```python
from build123d import *

# Parameters (mm, degrees)
SKETCH2_R           = 3.142219065
SKETCH2_W           = 25.3952265
SKETCH2_H           = 12.629529533
SKETCH2_R_2         = 3.175
SKETCH2_R_3         = 8.75000028
BOSS_EXTRUDE1_DEPTH = 80.000094
CUT_EXTRUDE2_DEPTH  = 179.822094
SKETCH6_R           = 6.35
SKETCH6_R_2         = 6.248785159
CUT_EXTRUDE6_DEPTH  = 41.402
BOSS_EXTRUDE4_START = 25.4
SKETCH6_10_R        = 6.35
SKETCH6_10_R_2      = 6.248785159
BOSS_EXTRUDE4_DEPTH = 25.4


with BuildPart() as part:
    # Sketch2 → Boss-Extrude1 (new body)
    with BuildSketch(Plane.XY):
        Polygon((0, 0), (0, 81.061351085), (0, 101.6), (-152.4, 101.6), (-152.4, 81.061351085), (-152.4, 0), align=None)
        with Locations((-126.984472284, 29.74542377)):
            Circle(SKETCH2_R, mode=Mode.SUBTRACT)
        with Locations((-76.249140265, 29.791740678)):
            Rectangle(SKETCH2_W, SKETCH2_H, mode=Mode.SUBTRACT)
        with Locations((-25.384472284, 29.74542377)):
            Circle(SKETCH2_R_2, mode=Mode.SUBTRACT)
        with Locations((-113.538, 81.061351085)):
            Circle(SKETCH2_R_3, mode=Mode.SUBTRACT)
        with Locations((-38.952133661, 81.061351085)):
            Circle(SKETCH2_R_3, mode=Mode.SUBTRACT)
    extrude(amount=BOSS_EXTRUDE1_DEPTH)

    # Sketch3 → Cut-Extrude2 (cut)
    with BuildSketch(Plane(origin=(0, 101.6, 0), x_dir=(1, 0, 0), z_dir=(0, 1, 0))):
        Polygon((-20.334810309, -6.35), (-20.334810309, -73.650094), (-76.2, -73.650094), (-132.170994975, -73.650094), (-132.170994975, -6.35), (-76.2, -6.35), align=None)
    extrude(amount=-CUT_EXTRUDE2_DEPTH, mode=Mode.SUBTRACT)

    # Sketch6 → Cut-Extrude6 (cut)
    with BuildSketch(Plane(origin=(0, 0, 73.650094), x_dir=(-1, 0, 0), z_dir=(0, 0, -1))):
        with Locations((76.041292075, 59.740546456)):
            Circle(SKETCH6_R)
        with Locations((76.2, 85.662840915)):
            Circle(SKETCH6_R_2)
    extrude(amount=-CUT_EXTRUDE6_DEPTH, mode=Mode.SUBTRACT)

    # Sketch6_10 → Boss-Extrude4 (add)
    with BuildSketch(Plane(origin=(0, 0, 73.650094), x_dir=(-1, 0, 0), z_dir=(0, 0, -1)).offset(BOSS_EXTRUDE4_START)):
        Polygon((76.2, 101.6), (63.397560696, 101.6), (63.397560696, 50.8), (88.685023454, 50.8), (88.685023454, 101.6), align=None)
        with Locations((76.041292075, 59.740546456)):
            Circle(SKETCH6_10_R, mode=Mode.SUBTRACT)
        with Locations((76.2, 85.662840915)):
            Circle(SKETCH6_10_R_2, mode=Mode.SUBTRACT)
    extrude(amount=-BOSS_EXTRUDE4_DEPTH)


solid = part.part
```
The listing builds one solid part. Answer for the finished solid, in the listing's coordinates (mm). A direction names the side the tool comes from. Coordinates: 2 decimals unless noted, no trailing zeros. Write each loop counter-clockwise with the first axis right and the second up, starting at its lowest first coordinate (ties: lowest second). Pieces come first, ordered by that corner, then holes. Notation, with made-up numbers: (-25, 71.25) - (-20, 71.25) arc R13 cw to (-20, 95.25) - close; hole circle Ø8 at (79, 19). An arc over 180 degrees is marked (long way). Return JSON: item names as keys, results as strings. Group by question number.
Q1. The part is cut by section A-A on z = 15.5. Write down the section's boundary in (x, y), and give its area (3 significant figures).
Q2. Find the intervals of material crossed by line 1 along X through (y, z) = (72.5, 60); line 2 along X through (y, z) = (81.5, 30); line 3 along Z through (x, y) = (-32.5, 44.5), in increasing order. Write a range as [from, to].
Q3. The part is cut by section C-C on x = -76.2. Write down the section's boundary in (y, z).
Q4. A flat-ended cylindrical pin translates along its axis: pin 1 Ø10 at (x, z) = (-77.5, 63.5) entering from -Y. Find the tip coordinate at first contact, or state that the pin passes through.
Q5. The part is cut by section D-D on z = 54.5. Write down the section's boundary in (x, y).
Q6. Which of the six approach directions +Z, -Z, +X, -X, +Y, -Y give full straight-line access (tool end or side, diameter ignored) to faces 3 (the flat face through (-76, 23.477, 3)), 4 (the flat face through (-88.685, 76, 61)), 5 (the cylindrical face through (-74.85, 79.56, 63.9))?
Q7. For a pull along X with two mould halves and no side action, classify faces 1 (the flat face through (-63.552, 30, 3)), 2 (the flat face through (-77, 52, 0)) as +X half, -X half, draft (parallel to the pull), parting line (faces both ways), or undercut.
Q8. The part is cut by section B-B on y = 40. Write down the section's boundary in (x, z).
Evaluation:
{
 "1": {"outline": "(-152.4, 0) - (-132.17, 0) - (-132.17, 101.6) - (-152.4, 101.6) - close; (-20.33, 0) - (0, 0) - (0, 101.6) - (-20.33, 101.6) - close", "area": "4,120 mm2"},
 "2": {"line 1": "x = [-152.4, -132.17], [-88.69, -63.4], [-20.33, 0]", "line 2": "x = [-152.4, -132.17], [-20.33, 0]", "line 3": "z = [0, 6.35], [73.65, 80]"},
 "3": {"outline": "(0, 0) - (23.48, 0) - (23.48, 6.35) - (0, 6.35) - close; (0, 73.65) - (23.48, 73.65) - (23.48, 80) - (0, 80) - close; (36.11, 0) - (101.6, 0) - (101.6, 6.35) - (36.11, 6.35) - close; (36.11, 73.65) - (50.8, 73.65) - (50.8, 48.25) - (53.39, 48.25) - (53.39, 80) - (36.11, 80) - close; (66.09, 48.25) - (79.41, 48.25) - (79.41, 80) - (66.09, 80) - close; (91.91, 48.25) - (101.6, 48.25) - (101.6, 80) - (91.91, 80) - close"},
 "4": {"pin 1": "stops at y = 50.8"},
 "5": {"outline": "(-152.4, 0) - (-132.17, 0) - (-132.17, 101.6) - (-152.4, 101.6) - close; (-88.69, 50.8) - (-63.4, 50.8) - (-63.4, 101.6) - (-88.69, 101.6) - close; (-20.33, 0) - (0, 0) - (0, 101.6) - (-20.33, 101.6) - close; hole circle Ø12.5 at (-76.2, 85.66); hole circle Ø12.7 at (-76.04, 59.74)"},
 "6": {"face 3": "+Z, -Z", "face 4": "+Y, -Y", "face 5": "+Z"},
 "7": {"face 1": "undercut", "face 2": "draft"},
 "8": {"outline": "(-152.4, 0) - (0, 0) - (0, 80) - (-152.4, 80) - close; hole (-132.17, 6.35) - (-20.33, 6.35) - (-20.33, 73.65) - (-132.17, 73.65) - close"}
}
